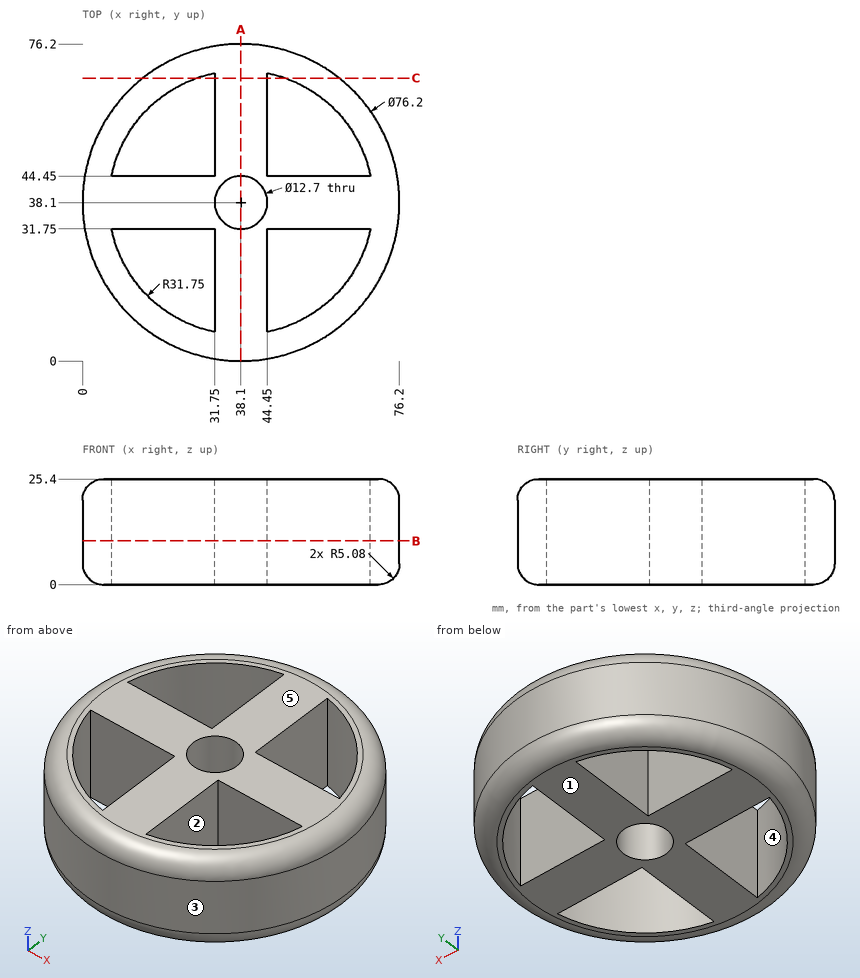
Drawing for the job (mm, zero at the part's lowest x, y, z). A direction names the side the tool comes from. Give positions to 0.01 mm unless a question says otherwise; leave off trailing zeros. Write each loop counter-clockwise with the first axis right and the second up, starting at its lowest first coordinate (ties: lowest second). Pieces come first, ordered by that corner, then holes. Notation, with made-up numbers: (63.5, -32.75) - (75.5, -32.75) arc R18 ccw to (75.5, -5.75) - close; hole circle Ø1 at (88, 3). An arc over 180 degrees is marked (long way). Answer as CSV lines item,"result".
Q1. Flat gauge pins, fed straight in: pin 1 Ø12.5 at (x, z) = (14, 11.5) entering from +Y; pin 2 Ø8 at (y, z) = (45, 22) entering from +X; pin 3 Ø12.5 at (x, z) = (15, 17) entering from -Y. Where does each tip first touch, or does it go through?
Result set:
pin 1,"y = 71.76"
pin 2,"x = 76.06"
pin 3,"y = 3.93"
Q2. Drill centre lines: line 1 (Y direction, x = 38.1, z = 14); line 2 (Y direction, x = 59.5, z = 6.25); line 3 (Y direction, x = 51, z = 10.75). Where is each one in solid material? Low to high. Write a range as from..to.
Result set:
line 1,"0..31.75, 44.45..76.2"
line 2,"6.58..14.65, 31.75..44.45, 61.55..69.62"
line 3,"2.25..9.09, 31.75..44.45, 67.11..73.95"
Q3. Band-saw the part on B-B (z = 10.5). Give the cut face in (x, y), and give its area (3 significant figures).
Result set:
outline,"circle Ø76.2 at (38.1, 38.1); hole (6.99, 31.75) arc R31.75 ccw to (31.75, 6.99) - (31.75, 31.75) - close; hole (6.99, 44.45) - (31.75, 44.45) - (31.75, 69.21) arc R31.75 ccw to start; hole circle Ø12.7 at (38.1, 38.1); hole (44.45, 6.99) arc R31.75 ccw to (69.21, 31.75) - (44.45, 31.75) - close; hole (44.45, 44.45) - (69.21, 44.45) arc R31.75 ccw to (44.45, 69.21) - close"
area,"2,710 mm²"
Q4. 3-axis set-ups, long thin cutter, end or side, ignore diameter. For the marked faces 1 and 2: which of +Z, -Z, +X, -X, +Y, -Y reach the whole face in a straight line?
Result set:
face 1,"-Z, +X, -X, +Y, -Y"
face 2,"+Z, -Z"
Q5. Pull direction X, two halves, no side cores. Call the marked faces 3, 4 and 5: released by +X, released by -X, zero draft, split by the parting line, or undercut.
Result set:
face 3,"split by the parting line"
face 4,"undercut"
face 5,"zero draft"
Q6. Band-saw the part on C-C (y = 68). State how many separate pieces and enclosed holes the cut face has, and give its area (3 significant figures).
Result set:
separate pieces,"3"
enclosed holes,"0"
area,"942 mm²"
Q7. Band-saw the part on A-A (x = 38.1). Give the cut face in (y, z), and give its area (3 significant figures).
Result set:
outline,"(0, 5.08) arc R5.08 ccw to (5.08, 0) - (31.75, 0) - (31.75, 25.4) - (5.08, 25.4) arc R5.08 ccw to (0, 20.32) - close; (44.45, 0) - (71.12, 0) arc R5.08 ccw to (76.2, 5.08) - (76.2, 20.32) arc R5.08 ccw to (71.12, 25.4) - (44.45, 25.4) - close"
area,"1,590 mm²"
